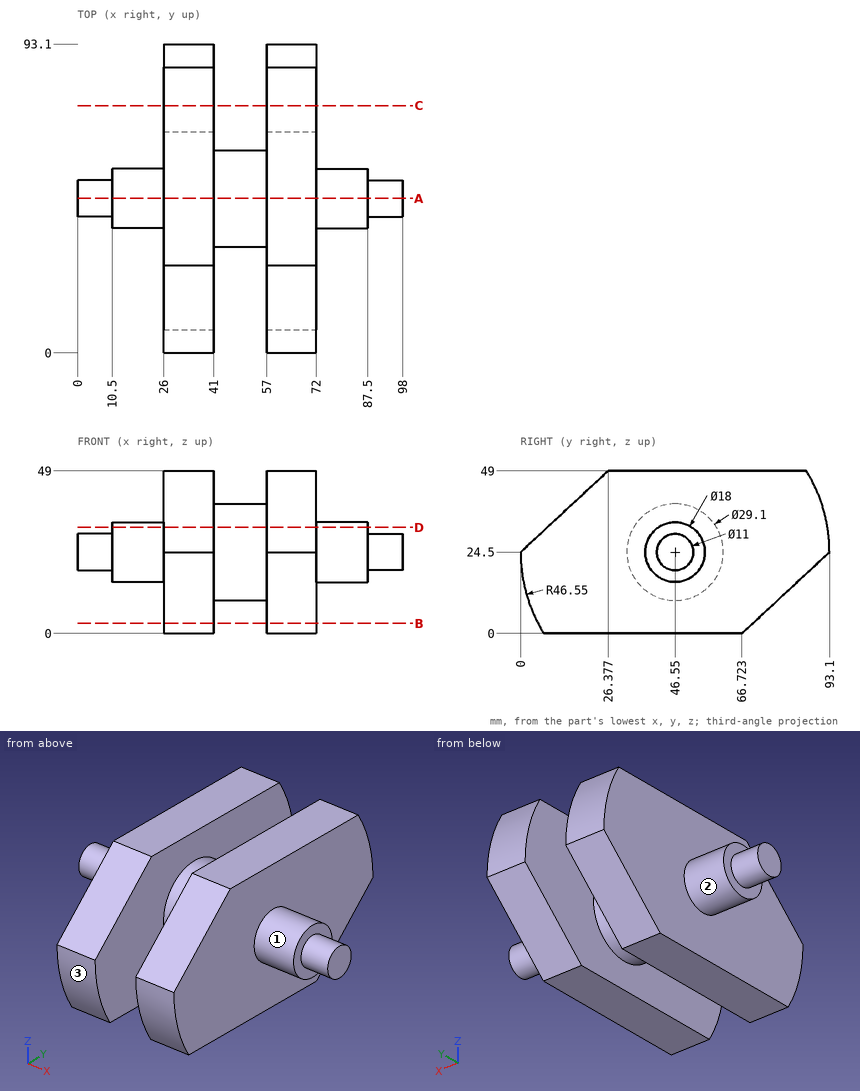
For this review, use the dimensioned drawing (mm, ordinates from the lowest corner) and the shaded views. A direction names the side the tool comes from. Give positions to 0.01 mm unless a question says otherwise; leave off trailing zeros. Write each loop counter-clockwise with the first axis right and the second up, starting at its lowest first coordinate (ties: lowest second). Pieces come first, ordered by that corner, then holes.
(1) Consider section A-A, the plane y = 46.55. Give the boundary of the cut face in (x, z), and give its area (3 significant figures).
(2) Tool access review of the marked faces 1, 2 and 3: name each direction out of +Z, -Z, +X, -X, +Y, -Y from which nothing blocks a thin tool from reaching the whole face with its end or side.
(3) For P1, Ø5, axis at x = 86.5, z = 22.5, coming from the +Y side; P2, Ø2, axis at y = 58.5, z = 13.5, coming from the -X side; P3, Ø10, axis at x = 36, z = 5.5, coming from the +Y side, all flat-tipped, find the tip position at first contact; note any pin that passes through.
(4) Consider section C-C, the plane y = 74.5. Give the boundary of the cut face in (x, z).
(5) Consider section B-B, the plane z = 3. Give the boundary of the cut face in (x, y), and give its area (3 significant figures).
(6) To check wall thickness, follow L1, parallel to X at y = 64.5, z = 13.5; L2, parallel to X at y = 37, z = 21.5; L3, parallel to Y at x = 24, z = 25. State the ranges of each line that lie inside material, in increasing order.
(7) Consider section D-D, the plane z = 32. Give the boundary of the cut face in (x, y) (1 decimal).
Returned:
1. outline: (0, 19) - (10.5, 19) - (10.5, 15.5) - (26, 15.5) - (26, 0) - (41, 0) - (41, 9.95) - (57, 9.95) - (57, 0) - (72, 0) - (72, 15.5) - (87.5, 15.5) - (87.5, 19) - (98, 19) - (98, 30) - (87.5, 30) - (87.5, 33.5) - (72, 33.5) - (72, 49) - (57, 49) - (57, 39.05) - (41, 39.05) - (41, 49) - (26, 49) - (26, 33.5) - (10.5, 33.5) - (10.5, 30) - (0, 30) - close
1. area: 2,720 mm2
2. face 1: +X
2. face 2: -X
2. face 3: -Z, +X, -X, -Y
3. P1: stops at y = 55.55
3. P2: stops at x = 26
3. P3: stops at y = 78.03
4. outline: (26, 7.22) - (41, 7.22) - (41, 49) - (26, 49) - close; (57, 7.22) - (72, 7.22) - (72, 49) - (57, 49) - close
5. outline: (26, 5.26) - (41, 5.26) - (41, 69.95) - (26, 69.95) - close; (57, 5.26) - (72, 5.26) - (72, 69.95) - (57, 69.95) - close
5. area: 1,940 mm2
6. L1: x = 26 to 41, 57 to 72
6. L2: x = 26 to 72
6. L3: y = 37.56 to 55.54
7. outline: (10.5, 41.6) - (26, 41.6) - (26, 8.1) - (41, 8.1) - (41, 34.1) - (57, 34.1) - (57, 8.1) - (72, 8.1) - (72, 41.6) - (87.5, 41.6) - (87.5, 51.5) - (72, 51.5) - (72, 92.5) - (57, 92.5) - (57, 59) - (41, 59) - (41, 92.5) - (26, 92.5) - (26, 51.5) - (10.5, 51.5) - close
